from build123d import *

# Parameters (mm, degrees)
ESQUISSE2_R             = 3.1
ENL_V_MAT_EXTRU_1_DEPTH = 21
ENL_V_MAT_EXTRU_2_DEPTH = 2
ESQUISSE4_R             = 2.6
ENL_V_MAT_EXTRU_3_DEPTH = 21
ESQUISSE5_R             = 4.25
ENL_V_MAT_EXTRU_4_DEPTH = 5.2
CONG_1_R                = 6


with BuildPart() as part:
    # Esquisse1 → Révolution1 (revolve)
    with BuildSketch(Plane.XY):
        Polygon((-40.55, 0), (-40.55, 12), (-47.55, 12), (-47.55, 20), (-65, 20), (-90, 20), (-90, 2), (-65, 2), (-65, 0), (-50.3, 0), (-50.3, 6), (-47.1, 6), (-47.1, 0), align=None)
    revolve(axis=Axis((0, 0, 0), (0, 1, 0)))

    # Esquisse2 → Enlèv. mat.-Extru.1 (cut, through all)
    with BuildSketch(Plane.XZ):
        with Locations((0, 58)):
            Circle(ESQUISSE2_R)
        with Locations((41.012193309, 41.012193309)):
            Circle(ESQUISSE2_R)
        with Locations((58, 0)):
            Circle(ESQUISSE2_R)
        with Locations((41.012193309, -41.012193309)):
            Circle(ESQUISSE2_R)
        with Locations((0, -58)):
            Circle(ESQUISSE2_R)
        with Locations((-41.012193309, -41.012193309)):
            Circle(ESQUISSE2_R)
        with Locations((-58, 0)):
            Circle(ESQUISSE2_R)
        with Locations((-41.012193309, 41.012193309)):
            Circle(ESQUISSE2_R)
    extrude(amount=-ENL_V_MAT_EXTRU_1_DEPTH, mode=Mode.SUBTRACT)

    # Esquisse3 → Enlèv. mat.-Extru.2 (cut)
    with BuildSketch(Plane(origin=(0, 20, 0), x_dir=(1, 0, 0), z_dir=(0, 1, 0))):
        Polygon((-52.810313666, 52.810313666), (-74.68506182, 0), (-52.810313666, -52.810313666), (0, -74.68506182), (52.810313666, -52.810313666), (74.68506182, 0), (52.810313666, 52.810313666), (0, 74.68506182), align=None)
    extrude(amount=-ENL_V_MAT_EXTRU_2_DEPTH, mode=Mode.SUBTRACT)

    # Esquisse4 → Enlèv. mat.-Extru.3 (cut, through all)
    with BuildSketch(Plane(origin=(0, 20, 0), x_dir=(1, 0, 0), z_dir=(0, 1, 0))):
        with Locations((0, 80)):
            Circle(ESQUISSE4_R)
        with Locations((56.568542495, 56.568542495)):
            Circle(ESQUISSE4_R)
        with Locations((80, 0)):
            Circle(ESQUISSE4_R)
        with Locations((56.568542495, -56.568542495)):
            Circle(ESQUISSE4_R)
        with Locations((0, -80)):
            Circle(ESQUISSE4_R)
        with Locations((-56.568542495, -56.568542495)):
            Circle(ESQUISSE4_R)
        with Locations((-80, 0)):
            Circle(ESQUISSE4_R)
        with Locations((-56.568542495, 56.568542495)):
            Circle(ESQUISSE4_R)
    extrude(amount=-ENL_V_MAT_EXTRU_3_DEPTH, mode=Mode.SUBTRACT)

    # Esquisse5 → Enlèv. mat.-Extru.4 (cut)
    with BuildSketch(Plane(origin=(0, 20, 0), x_dir=(1, 0, 0), z_dir=(0, 1, 0))):
        with Locations((0, 80)):
            Circle(ESQUISSE5_R)
        with Locations((56.568542495, 56.568542495)):
            Circle(ESQUISSE5_R)
        with Locations((80, 0)):
            Circle(ESQUISSE5_R)
        with Locations((56.568542495, -56.568542495)):
            Circle(ESQUISSE5_R)
        with Locations((0, -80)):
            Circle(ESQUISSE5_R)
        with Locations((-56.568542495, -56.568542495)):
            Circle(ESQUISSE5_R)
        with Locations((-80, 0)):
            Circle(ESQUISSE5_R)
        with Locations((-56.568542495, 56.568542495)):
            Circle(ESQUISSE5_R)
    extrude(amount=-ENL_V_MAT_EXTRU_4_DEPTH, mode=Mode.SUBTRACT)

    # Congé1
    cong_1_edges = [part.edges().sort_by_distance(p)[0] for p in [
        (-52.810313666, 19, 52.810313666),
        (-74.68506182, 19, 0),
        (-52.810313666, 19, -52.810313666),
        (0, 19, -74.68506182),
        (52.810313666, 19, -52.810313666),
        (74.68506182, 19, 0),
        (52.810313666, 19, 52.810313666),
        (0, 19, 74.68506182),
    ]]
    fillet(cong_1_edges, radius=CONG_1_R)


solid = part.part
Here's how the part is built. I have some questions about the finished solid (model axes, mm). A direction names the side the tool comes from. Coordinates: 2 decimals unless noted, no trailing zeros. Loops run counter-clockwise (first coordinate to the right, second up) from the corner with the lowest first, then second, coordinate; pieces in that order, holes last.
1. I need wall thicknesses on L1, parallel to Z at x = 0, y = 13.5; L2, parallel to Z at x = 0, y = 16.85; L3, parallel to Z at x = -58, y = 11.25. Which ranges of each line are inside material? Lowest first, please.
2. For faces 1 (the flat face through (26.068, 19.014, 63.887)), 2 (the cylindrical face through (-54.089, 8.49, 55.788)), 3 (the cylindrical face through (-62, 0.99, 19.52)), which set-ups out of +Z, -Z, +X, -X, +Y, -Y let a thin tool reach every point of the face, with its end or its side?
3. Imagine slicing it at A-A, the plane z = 11. Please give me the cut outline in (x, y).
4. Imagine slicing it at C-C, the plane x = 0. Count the separate pieces of the cut face and the enclosed holes in it, and give its area (3 significant figures).
5. If we mould it in two halves opening along X, with no side actions, what happens to faces 4 (the cylindrical face through (-41.53, 10.874, -79.845)), 5 (the cylindrical face through (59.05, 8.49, -57.35)), 6 (the flat face through (48.5, 0, -14.1)), 7 (the cylindrical face through (-0.404, 8.874, -54.926))? For each: pulls with the +X half, pulls with the -X half, needs draft (parallel to the pull), parting line crosses it, or undercut.
6. Imagine slicing it at B-B, the plane x = -80. Please give me the cut outline in (y, z), and give its area (3 significant figures).
7. Imagine slicing it at D-D, the plane z = -11.5. Please give me the cut outline in (x, y).
8. For P1, Ø7, axis at x = 41.01, z = 41.01, coming from the +Y side; P2, Ø1, axis at y = 17.5, z = 12, coming from the +X side; P3, Ø10, axis at x = 58.5, z = 39, coming from the -Y side; P4, Ø5, axis at x = 56.57, z = 56.57, coming from the -Y side, each with a flat end and sliding along its axis, tell me the tip position at first contact or that it passes through.
Taken from the geometry:
1. L1: z = -90 to -82.6, -77.4 to -61.1, -54.9 to -47.55, 47.55 to 54.9, 61.1 to 77.4, 82.6 to 90
1. L2: z = -90 to -84.25, -75.75 to -61.1, -54.9 to -47.55, 47.55 to 54.9, 61.1 to 75.75, 84.25 to 90
1. L3: z = -68.82 to -58.74, -54.4 to -3.1, 3.1 to 54.4, 58.74 to 68.82
2. face 1: +Y
2. face 2: +Y, -Y
2. face 3: -Y
3. outline: (-89.33, 2) - (-64.06, 2) - (-64.06, 0) - (-49.08, 0) - (-49.08, 6) - (-45.8, 6) - (-45.8, 0) - (-39.03, 0) - (-39.03, 12) - (-46.26, 12) - (-46.26, 18) - (-70.13, 18) - (-70.13, 20) - (-89.33, 20) - close; (39.03, 0) - (45.8, 0) - (45.8, 6) - (49.08, 6) - (49.08, 0) - (64.06, 0) - (64.06, 2) - (89.33, 2) - (89.33, 20) - (70.13, 20) - (70.13, 18) - (46.26, 18) - (46.26, 12) - (39.03, 12) - close
4. separate pieces: 6
4. enclosed holes: 0
4. area: 1,180 mm2
5. face 4: parting line crosses it
5. face 5: undercut
5. face 6: needs draft
5. face 7: undercut
6. outline: (2, -41.23) - (20, -41.23) - (20, -4.25) - (14.8, -4.25) - (14.8, -2.6) - (2, -2.6) - close; (2, 2.6) - (14.8, 2.6) - (14.8, 4.25) - (20, 4.25) - (20, 41.23) - (2, 41.23) - close
6. area: 1,370 mm2
7. outline: (-89.26, 2) - (-63.97, 2) - (-63.97, 0) - (-48.97, 0) - (-48.97, 6) - (-45.67, 6) - (-45.67, 0) - (-38.89, 0) - (-38.89, 12) - (-46.14, 12) - (-46.14, 18) - (-69.92, 18) - (-69.92, 20) - (-89.26, 20) - close; (38.89, 0) - (45.67, 0) - (45.67, 6) - (48.97, 6) - (48.97, 0) - (63.97, 0) - (63.97, 2) - (89.26, 2) - (89.26, 20) - (69.92, 20) - (69.92, 18) - (46.14, 18) - (46.14, 12) - (38.89, 12) - close
8. P1: stops at y = 18
8. P2: stops at x = 89.26
8. P3: stops at y = 2
8. P4: passes through
